Design review of the part built by this model. Coordinates are the model's own, in mm. Face numbers are marked on the shaded views. A direction names the side the tool comes from. Coordinates: 2 decimals unless noted, no trailing zeros. Write each loop counter-clockwise with the first axis right and the second up, starting at its lowest first coordinate (ties: lowest second). Pieces come first, ordered by that corner, then holes.
Q1. Take a section at C-C, the plane z = 1.1. State how many separate pieces and enclosed holes the cut face has, plus the area to 3 significant figures.
Q2. For L1, parallel to X at y = -27, z = 1.7; L2, parallel to Y at x = 0, z = 4.05; L3, parallel to X at y = -34, z = 1.6, list the stretches that pass through material, from the lowest coordinate up.
Q3. Take a section at D-D, the plane y = -11.5. Write out the cut boundary in (x, z), plus the area to 3 significant figures.
Q4. For the marked faces 1, 2 and 3, list the 3-axis set-ups (+Z, -Z, +X, -X, +Y, -Y) from which the entire face can be reached by the end or side of a thin tool; tool diameter is ignored.
Q5. For pin 1 Ø1 at (x, z) = (-36.5, 3) entering from +Y; pin 2 Ø2.5 at (x, z) = (-2, 2.5) entering from +Y; pin 3 Ø2.5 at (x, z) = (28, 2.5) entering from -Y, all flat-tipped, find the tip position at first contact; note any pin that passes through.
Q6. The part is to be moulded in two halves that separate along Y. For the marked faces 4, 5 and 6, say which applies: released by +Y, released by -Y, zero draft, split by the parting line, or undercut.
Q7. Take a section at A-A, the plane y = 0. Write out the cut boundary in (x, z), plus the area to 4 significant figures.
Q8. Take a section at B-B, the plane x = 0. Write out the cut boundary in (y, z), plus the area to 4 significant figures.
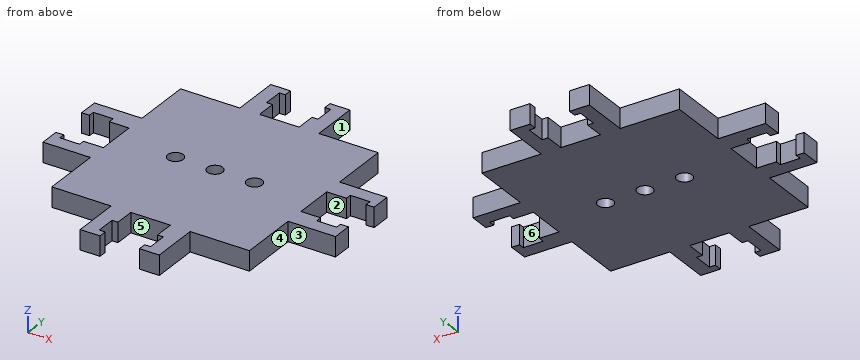
from build123d import *

# Parameters (mm, degrees)
ESQUISSE1_R        = 1.95
BOSS_EXTRU_1_DEPTH = 5


with BuildPart() as part:
    # Esquisse1 → Boss.-Extru.1 (new body)
    with BuildSketch(Plane.XY):
        Polygon((-10, 25), (-25, 25), (-25, 10), (-30, 10), (-37, 10), (-37, 5), (-35, 5), (-35, 6.5), (-30, 6.5), (-30, 5), (-25, 5), (-25, 0), (-25, -5), (-30, -5), (-30, -6.5), (-35, -6.5), (-35, -5), (-37, -5), (-37, -10), (-30, -10), (-25, -10), (-25, -25), (-10, -25), (-10, -30), (-10, -37), (-5, -37), (-5, -35), (-6.5, -35), (-6.5, -30), (-5, -30), (-5, -25), (0, -25), (5, -25), (5, -30), (6.5, -30), (6.5, -35), (5, -35), (5, -37), (10, -37), (10, -30), (10, -25), (25, -25), (25, -10), (30, -10), (37, -10), (37, -5), (35, -5), (35, -6.5), (30, -6.5), (30, -5), (25, -5), (25, 0), (25, 5), (30, 5), (30, 6.5), (35, 6.5), (35, 5), (37, 5), (37, 10), (30, 10), (25, 10), (25, 25), (10, 25), (10, 30), (10, 37), (5, 37), (5, 35), (6.5, 35), (6.5, 30), (5, 30), (5, 25), (0, 25), (-5, 25), (-5, 30), (-6.5, 30), (-6.5, 35), (-5, 35), (-5, 37), (-10, 37), (-10, 30), align=None)
        with Locations((-10, 0)):
            Circle(ESQUISSE1_R, mode=Mode.SUBTRACT)
        Circle(ESQUISSE1_R, mode=Mode.SUBTRACT)
        with Locations((10, 0)):
            Circle(ESQUISSE1_R, mode=Mode.SUBTRACT)
    extrude(amount=BOSS_EXTRU_1_DEPTH)


solid = part.part
Responses:
1. separate pieces: 1
1. enclosed holes: 3
1. area: 2,880 mm2
2. L1: x = -10 to -5, 5 to 10
2. L2: y = -25 to -1.95, 1.95 to 25
2. L3: x = -10 to -6.5, 6.5 to 10
3. outline: (-25, 0) - (25, 0) - (25, 5) - (-25, 5) - close
3. area: 250 mm2
4. face 1: +Z, -Z, +X, +Y
4. face 2: +Z, -Z, +X
4. face 3: +Z, -Z, +X, -Y
5. pin 1: stops at y = 10
5. pin 2: stops at y = 25
5. pin 3: stops at y = -10
6. face 4: zero draft
6. face 5: released by -Y
6. face 6: undercut
7. outline: (-25, 0) - (-11.95, 0) - (-11.95, 5) - (-25, 5) - close; (-8.05, 0) - (-1.95, 0) - (-1.95, 5) - (-8.05, 5) - close; (1.95, 0) - (8.05, 0) - (8.05, 5) - (1.95, 5) - close; (11.95, 0) - (25, 0) - (25, 5) - (11.95, 5) - close
7. area: 191.5 mm2
8. outline: (-25, 0) - (-1.95, 0) - (-1.95, 5) - (-25, 5) - close; (1.95, 0) - (25, 0) - (25, 5) - (1.95, 5) - close
8. area: 230.5 mm2
